Autodesk Inventor part; units mm, degrees
ref_plane "Work Plane1" through (5.5499, 0, 34.925) normal (1, 0, 0) x (0, 1, 0)
ref_plane "XZ Plane" through (0, 0, 0) normal (0, 1, 0) x (-1, 0, 0)
ref_plane "XY Plane" through (0, 0, 0) normal (0, 0, 1) x (1, 0, 0)
sketch "Sketch1" plane through (0, 0, 0) normal (1, 0, 0) x (0, 1, 0)
  line L0 (-5.5499, 0) -> (-5.5499, 69.85)
  line L1 (0, 0) -> (-5.5499, 0)
  line L2 (-3.0543, 69.85) -> (-5.5499, 69.85)
  line L3 (0, 73.9634) -> (0, 0)
  line L4 (-3.0543, 73.9634) -> (-3.0543, 69.85)
  line L5 (-3.0543, 73.9634) -> (0, 73.9634)
  dimension "d1" = 73.9634
  dimension "d3" = 5.5499
  dimension "d4" = 69.85
  dimension "d6" = 4.1134
  dimension "d8" = 2.4956
revolve "Revolution1" add sketch "Sketch1" angle 360 about axis through (0, 0, 73.9634) along (0, 0, -1)
sketch "Sketch2" plane through (0, 0, 0) normal (1, 0, 0) x (0, 1, 0)
  line L0 (3.0543, 73.9634) -> (-3.0543, 73.9634) construction
  arc A0 (5.9944, 79.121) -> (-5.9944, 79.121) centre (0, 79.121) ccw
  line L1 (5.5499, 69.85) -> (-5.5499, 69.85)
  line L2 (5.9944, 79.121) -> (-5.9944, 79.121)
  point P0 (0, 0)
  point P1 (0, 73.9634)
  point P2 (0, 69.85)
  dimension "d12" = 11.9888
  dimension "d21" = 5.1576
  dimension "d22" = 9.271
  dimension "d23" = 6.1087
revolve "Revolution2" add sketch "Sketch2" angle 360 about axis through (0, 5.9944, 79.121) along (0, -1, 0)
chamfer "Chamfer1" distance 0.9652 angle 45 2 edges at (0, 5.5499, 69.85) (0, 5.5499, 0)
ref_plane "Work Plane1" through (5.5499, 0, 34.925) normal (1, 0, 0) x (0, 1, 0)
sketch "Sketch3" plane through (5.5499, 0, 34.925) normal (1, 0, 0) x (0, 1, 0)
  point P0 (0, -34.925)
  point P1 (0, -30.099)
  dimension "d30" = 4.826
hole "Hole1" at (5.5499, 0, 4.826) direction (-1, 0, 0) diameter 4.8006 end through all
properties part number "Ball_2"
Read the model definition and answer for the solid it produces. Units are mm, in the model's axes. A direction names the side the tool comes from. Give positions to 0.01 mm unless a question says otherwise; leave off trailing zeros. Write each loop counter-clockwise with the first axis right and the second up, starting at its lowest first coordinate (ties: lowest second). Pieces come first, ordered by that corner, then holes. Notation, with made-up numbers: (-16, 4) - (35, 4) arc R11 ccw to (35, 25) - close; hole circle Ø5 at (12, -11). An arc over 180 degrees is marked (long way). Use CSV: the item, a comma, the result in double quotes. Start each with the question number.
(1) For faces 1 (the cylindrical face through (-2.126, -5.127, 35.4)), 2 (the cylindrical face through (-0.078, -0.721, 2.537)), determine the directions among +Z, -Z, +X, -X, +Y, -Y from which every point of the face is accessible in a straight line to the end or side of a thin tool.
(2) Determine the mould class of faces 3 (the cylindrical face through (-0.917, -2.913, 71.878)), 4 (the flat face through (0, 0, 0)) for opening direction Z: +Z half, -Z half, draft (parallel to the pull), parting line (faces both ways), or undercut.
(3) Consider line 1 along Z through (x, y) = (-0.25, 0); line 2 along Z through (x, y) = (-3.75, 2); line 3 along Z through (x, y) = (5.25, 1.5). Determine where each line is inside the solid, lowest interval first.
(4) Find section A-A (y = 0). Give the vertices of the cut face in (x, z).
(5) Find section B-B (z = 13). Give the vertices of the cut face in (x, y).
(6) Given P1, Ø3, axis at y = -1, z = 61.5, coming from the -X side; P2, Ø4, axis at y = -3.5, z = 45, coming from the +X side; P3, Ø4, axis at x = -3, y = 3.5, coming from the +Z side, each flat-ended and moving along its own axis, determine where each tip first touches the part or whether it passes through.
Findings below:
1,face 1,"-Z"
1,face 2,"+X, -X"
2,face 3,"undercut"
2,face 4,"-Z half"
3,line 1,"0 to 2.43, 7.23 to 85.11"
3,line 2,"0 to 3.5, 6.15 to 69.85, 74.89 to 83.35"
3,line 3,"0.88 to 2.95, 6.7 to 68.97, 76.65 to 81.59"
4,outline,"(-5.55, 0.97) - (-4.58, 0) - (4.58, 0) - (5.55, 0.97) - (5.55, 2.43) - (-5.55, 2.43) - close; (-5.55, 7.23) - (5.55, 7.23) - (5.55, 68.88) - (4.58, 69.85) - (3.05, 69.85) - (3.05, 73.96) arc R5.99 ccw (long way) to (-3.05, 73.96) - (-3.05, 69.85) - (-4.58, 69.85) - (-5.55, 68.88) - close"
5,outline,"circle Ø11.1 at (0, 0)"
6,P1,"x = -5.55"
6,P2,"x = 5.34"
6,P3,"z = 84.52"
